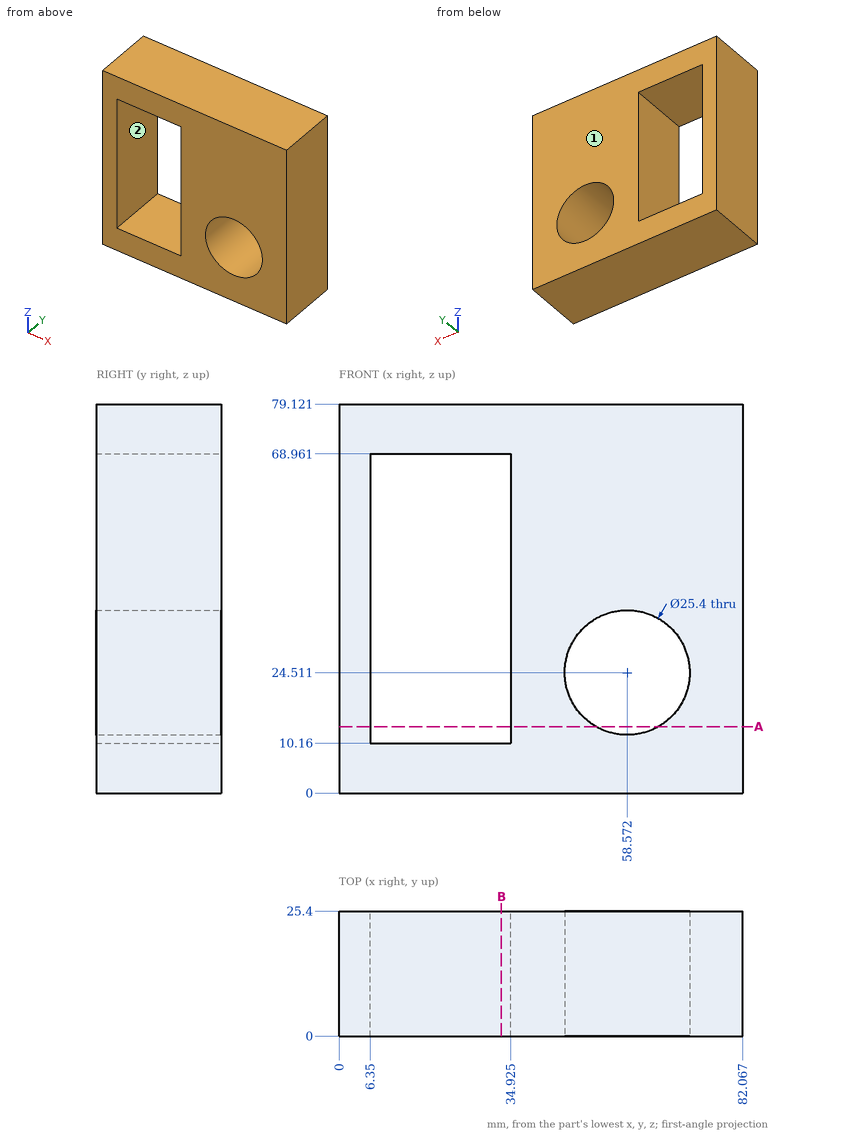
For this review, use the dimensioned drawing (mm, ordinates from the lowest corner) and the shaded views. A direction names the side the tool comes from. Give positions to 0.01 mm unless a question says otherwise; leave off trailing zeros. Write each loop counter-clockwise with the first axis right and the second up, starting at its lowest first coordinate (ties: lowest second). Pieces come first, ordered by that corner, then holes. Notation, with made-up numbers: M 78.25,82 L 117.25,82 A12 ccw 117.25,87 Z; hole C -14.75,-29.75 d3. An arc over 180 degrees is marked long. Write item = value, one per line. Start each with the question number.
Q1. For line 1 (Z direction, x = 10.5, y = 13.25); line 2 (Z direction, x = 65.5, y = 1.5) (1 decimal), list the stretches that pass through material, from the lowest coordinate up.
Q2. Machinability: for the marked faces 1 and 2, which of the approach directions +Z, -Z, +X, -X, +Y, -Y give a long, thin tool a straight path to every point of the face, cutting with its end or side? Answer none if there is none.
Q3. We need section B-B (x = 33). State the section outline as (y, z) points.
Q4. Clearance check with a flat-ended pin moving along its axis: pin 1 (12.5 mm diameter, centred on x = 17, y = 18.5, fed in from -Z). State where the tip first meets the part, or that it passes through.
Q5. We need section A-A (z = 13.5). Give the number of separate pieces and of enclosed holes in the cut face, plus the area to 3 significant figures.
Result set:
q1.line_1 = 0 to 10.16, 68.96 to 79.12
q1.line_2 = 0 to 13.9, 35.2 to 79.1
q2.face_1 = +Z, -Z, +X, -X, +Y
q2.face_2 = +Y, -Y
q3.outline = M 0,0 L 25.4,0 L 25.4,10.16 L 0,10.16 Z; M 0,68.96 L 25.4,68.96 L 25.4,79.12 L 0,79.12 Z
q4.pin_1 = 0
q5.separate_pieces = 3
q5.enclosed_holes = 0
q5.area = 1,040 mm2
